from build123d import *

# Parameters (mm, degrees)
SKETCH1_R           = 1.8
SKETCH1_R_2         = 5.3
BOSS_EXTRUDE1_DEPTH = 10
SKETCH2_R           = 3
CUT_EXTRUDE1_DEPTH  = 3.5
CUT_EXTRUDE2_START  = -5
CUT_EXTRUDE2_DEPTH  = 5


with BuildPart() as part:
    # Sketch1 → Boss-Extrude1 (new body)
    with BuildSketch(Plane.XY):
        with BuildLine():
            Line((0, 5), (60, 5))
            ThreePointArc((60, 5), (66.5, -1.5), (60, -8))
            Line((60, -8), (24.5, -8))
            Line((24.5, -8), (24.5, -33))
            ThreePointArc((24.5, -33), (21.571067812, -40.071067812), (14.5, -43))
            Line((14.5, -43), (-24, -43))
            ThreePointArc((-24, -43), (-32.485281374, -39.485281374), (-36, -31))
            ThreePointArc((-36, -31), (-31, -26), (-26, -31))
            Line((-26, -31), (-10, -31))
            ThreePointArc((-10, -31), (-2.928932188, -28.071067812), (0, -21))
            Line((0, -21), (0, -5))
            ThreePointArc((0, -5), (-5, 0), (0, 5))
        make_face()
        Circle(SKETCH1_R, mode=Mode.SUBTRACT)
        with Locations((14.5, -33)):
            Circle(SKETCH1_R_2, mode=Mode.SUBTRACT)
        with Locations((14.5, -11)):
            Circle(SKETCH1_R_2, mode=Mode.SUBTRACT)
        with Locations((0, -31)):
            Circle(SKETCH1_R, mode=Mode.SUBTRACT)
        with Locations((-31, -31)):
            Circle(SKETCH1_R, mode=Mode.SUBTRACT)
        with BuildLine():
            Line((60, -4.2), (40, -4.2))
            ThreePointArc((40, -4.2), (38.3, -2.5), (40, -0.8))
            Line((40, -0.8), (60, -0.8))
            ThreePointArc((60, -0.8), (61.7, -2.5), (60, -4.2))
        make_face(mode=Mode.SUBTRACT)
    extrude(amount=BOSS_EXTRUDE1_DEPTH)

    # Sketch2 → Cut-Extrude1 (cut)
    with BuildSketch(Plane.XY.offset(10)):
        with Locations((-31, -31)):
            Circle(SKETCH2_R)
        with Locations((0, -31)):
            Circle(SKETCH2_R)
        Circle(SKETCH2_R)
    extrude(amount=-CUT_EXTRUDE1_DEPTH, mode=Mode.SUBTRACT)

    # Sketch3 → Cut-Extrude2 (cut)
    with BuildSketch(Plane.XY.offset(10).offset(CUT_EXTRUDE2_START)):
        with BuildLine():
            Line((24.5, -8), (24.5, 0))
            ThreePointArc((24.5, 0), (23.035533906, 3.535533906), (19.5, 5))
            Line((19.5, 5), (60, 5))
            ThreePointArc((60, 5), (66.5, -1.5), (60, -8))
            Line((60, -8), (24.5, -8))
        make_face()
    extrude(amount=CUT_EXTRUDE2_DEPTH, mode=Mode.SUBTRACT)


solid = part.part
For this review, take the finished solid that the model builds, in its own axes (mm). A direction names the side the tool comes from. Give positions to 0.01 mm unless a question says otherwise; leave off trailing zeros. Loops run counter-clockwise (first coordinate to the right, second up) from the corner with the lowest first, then second, coordinate; pieces in that order, holes last. Notation, with made-up numbers: M 52,88.25 L 85,88.25 A14 cw 85,109.25 Z; hole C 12,87.5 d4. An arc over 180 degrees is marked long. Answer as a JSON object with one key per item and string values. Group by question number.
Q1. Add section C-C on x = 29. Give the boundary of the cut face in (y, z).
Q2. For probe 1 along Y at (x, z) = (14.5, 2.75); probe 2 along Y at (x, z) = (-2, 1.25); probe 3 along Y at (x, z) = (-31, 5.25), list the stretches that pass through material, from the lowest coordinate up. Write a range as [from, to].
Q3. Mouldability with a two-part tool opening along X and no side actions: class faces 6 (the flat face through (50, -0.8, 2)), 7 (the flat face through (-4, -43, 5)), 8 (the cylindrical face through (66.5, -1.4, 2.5)), 9 (the cylindrical face through (-34, -31, 8)) as +X half, -X half, draft (parallel to the pull), parting line (faces both ways), or undercut.
Q4. Add section B-B on z = 2. Give the boundary of the cut face in (x, y), and give its area (3 significant figures).
Q5. Add section D-D on y = -18. Give the boundary of the cut face in (x, z).
Q6. Tool access review of faces 1 (the cylindrical face through (-3, 0, 8)), 2 (the cylindrical face through (23.07, 3.5, 7.46)), 3 (the cylindrical face through (38.3, -2.5, 2.5)), 4 (the flat face through (0, -13, 5)), 5 (the flat face through (42, -8, 2)): name each direction out of +Z, -Z, +X, -X, +Y, -Y from which nothing blocks a thin tool from reaching the whole face with its end or side.
Q7. Insertion check: P1, Ø1.8, axis at x = -32, y = -31, coming from the +Z side; P2, Ø1.5, axis at x = 43.5, z = 2, coming from the -Y side; P3, Ø12, axis at x = 53, y = 0, coming from the +Z side. Each pin has a flat end and moves straight along its axis. Give the tip position at first contact, or say it passes through.
Q8. Add section A-A on x = 59. Give the boundary of the cut face in (y, z), and give its area (3 significant figures).
Checked values:
{
 "1": {"outline": "M -8,0 L 5,0 L 5,5 L -8,5 Z"},
 "2": {"probe 1": "[-43, -38.3], [-27.7, -16.3], [-5.7, 5]", "probe 2": "[-43, -27], [-4.58, 4.58]", "probe 3": "[-40.75, -32.8], [-29.2, -26]"},
 "3": {"face 6": "undercut", "face 7": "draft", "face 8": "+X half", "face 9": "undercut"},
 "4": {"outline": "M -36,-31 A12 ccw -24,-43 L 14.5,-43 A10 ccw 24.5,-33 L 24.5,-8 L 60,-8 A6.5 ccw 60,5 L 0,5 A5 ccw 0,-5 L 0,-21 A10 cw -10,-31 L -26,-31 A5 ccw Z; hole C -31,-31 d3.6; hole C 0,-31 d3.6; hole C 0,0 d3.6; hole C 14.5,-33 d10.6; hole C 14.5,-11 d10.6; hole M 40,-4.2 L 60,-4.2 A1.7 ccw 60,-0.8 L 40,-0.8 A1.7 ccw Z", "area": "1,900 mm²"},
 "5": {"outline": "M 0,0 L 24.5,0 L 24.5,10 L 0,10 Z"},
 "6": {"face 1": "+Z", "face 2": "+Z, +X, +Y", "face 3": "+Z, -Z", "face 4": "+Z, -Z, -X", "face 5": "+Z, -Z, +X, -Y"},
 "7": {"P1": "z = 6.5", "P2": "y = -8", "P3": "z = 5"},
 "8": {"outline": "M -8,0 L -4.2,0 L -4.2,5 L -8,5 Z; M -0.8,0 L 5,0 L 5,5 L -0.8,5 Z", "area": "48.0 mm²"}
}
